Build history of the part. All positions in model axes, mm. Face numbers are marked on the shaded views. A direction names the side the tool comes from. Round coordinates to 2 decimals unless told otherwise and drop trailing zeros. Order: outer loops, then holes, each group sorted by start corner. A loop starts at its lowest first (then second) coordinate and runs counter-clockwise, first axis right, second up. Notation, with made-up numbers: (59, 78.25) -> (66, 78.25) arc R18 ccw to (66, 101.25) -> close; hole circle Ø6 at (-22, 32). An arc over 180 degrees is marked (long way). Write item = value, one per line.
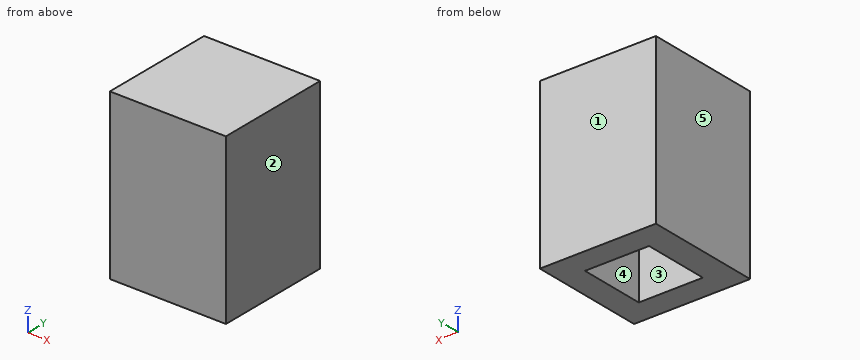
Autodesk Fusion 360 part; units mm, degrees
sketch "Sketch1" plane through (0, 0, 0) normal (0, 0, 1) x (1, 0, 0)
  line L0 (0, 0) -> (14, 0)
  line L1 (14, 0) -> (14, 14)
  line L2 (14, 14) -> (0, 14)
  line L3 (0, 14) -> (0, 0)
  line L4 (11, 11) -> (3.2653, 11)
  line L5 (3.2653, 11) -> (3.2653, 2.9996)
  line L6 (3.2653, 2.9996) -> (11, 2.9996)
  line L7 (11, 2.9996) -> (11, 11)
  line L8 (11, 11) -> (3.2653, 2.9996) construction
  line L9 (3.2653, 11) -> (11, 2.9996) construction
  point P0 (7.1326, 6.9998)
extrude "Extrude1" add sketch "Sketch1" along normal blind 20 contours L0 L1 L2 L3 | L4 L5 L6 L7
extrude "Extrude2" cut sketch "Sketch1" along normal blind 19 contours L4 L5 L6 L7
Q1. Cut at B-B, the plane x = 7. List the corners of the cut face in (y, z), and give its area (3 significant figures).
Check values:
outline = (0, 0) -> (3, 0) -> (3, 19) -> (11, 19) -> (11, 0) -> (14, 0) -> (14, 20) -> (0, 20) -> close
area = 128 mm²
Q2. Cut at C-C, the plane y = 7.75. List the corners of the cut face in (x, z).
Check values:
outline = (0, 0) -> (3.27, 0) -> (3.27, 19) -> (11, 19) -> (11, 0) -> (14, 0) -> (14, 20) -> (0, 20) -> close
Q3. Flat gauge pin, fed straight in: pin 1 (2.5 mm diameter, centred on x = 7, y = 7, fed in from -Z). Where does the tip first touch, or does it go through?
Check values:
pin_1 = 19
Q4. Which spindle directions (+Z, -Z, +X, -X, +Y, -Y) get a long thin tool onto all of the face, cutting with end or side? Do the marked faces 4 and 5. Say none if no direction does.
Check values:
face_4 = -Z
face_5 = +Z, -Z, -X, +Y, -Y
Q5. Cut at A-A, the plane z = 9.25. List the corners of the cut face in (x, y), and give its area (3 significant figures).
Check values:
outline = (0, 0) -> (14, 0) -> (14, 14) -> (0, 14) -> close; hole (3.27, 3) -> (11, 3) -> (11, 11) -> (3.27, 11) -> close
area = 134 mm²
Q6. Probe probe 1 along X at (y, z) = (10.75, 7.25); probe 2 along Y at (x, z) = (10.5, 3.25); probe 3 along Z at (x, y) = (3.5, 7). List the from-to ranges inside material, lowest first.
Check values:
probe_1 = 0 to 3.27, 11 to 14
probe_2 = 0 to 3, 11 to 14
probe_3 = 19 to 20
Q7. Mould opens along Y. For the marked faces 1, 2 and 3 say: released by +Y, released by -Y, zero draft, split by the parting line, or undercut.
Check values:
face_1 = released by +Y
face_2 = zero draft
face_3 = undercut
